from build123d import *

# Parameters (mm, degrees)
F1_DEPTH = 3.2


with BuildPart() as f1:
    # F0 (on Front) → F1 (new body)
    with BuildSketch(Plane.XZ):
        with BuildLine():
            Line((30.850063, 1.770954), (-56.149937, 1.770954))
            ThreePointArc((-56.149937, 1.770954), (-58.271257, 0.892275), (-59.149937, -1.229046))
            Line((-59.149937, -1.229046), (-59.149937, -16.129046))
            ThreePointArc((-59.149937, -16.129046), (-58.271257, -18.250366), (-56.149937, -19.129046))
            Line((-56.149937, -19.129046), (30.850063, -19.129046))
            ThreePointArc((30.850063, -19.129046), (32.971384, -18.250366), (33.850063, -16.129046))
            Line((33.850063, -16.129046), (33.850063, -1.229046))
            ThreePointArc((33.850063, -1.229046), (32.971384, 0.892275), (30.850063, 1.770954))
        make_face()
        Polygon((-56.249937, -16.129046), (-56.249937, -14.429046), (23.450063, -14.429046), (23.450063, -12.929046), (28.450063, -12.929046), (28.450063, -14.429046), (30.950063, -14.429046), (30.950063, -16.129046), align=None, mode=Mode.SUBTRACT)
    extrude(amount=F1_DEPTH)


solid = f1.part
The listing builds one solid part. Answer for the finished solid, in the listing's coordinates (mm). A direction names the side the tool comes from. Coordinates: 2 decimals unless noted, no trailing zeros. Order: outer loops, then holes, each group sorted by start corner. A loop starts at its lowest first (then second) coordinate and runs counter-clockwise, first axis right, second up. Notation, with made-up numbers: M 30.5,62 L 63.5,62 A11 ccw 63.5,72 Z; hole C 89,0.25 d7. An arc over 180 degrees is marked long. Use CSV: the item, a comma, the result in double quotes.
Q1. Section A-A (x = -26) is taken. Determine the outline of the cut face in (y, z).
Here are the results:
outline,"M -3.2,-19.13 L 0,-19.13 L 0,-16.13 L -3.2,-16.13 Z; M -3.2,-14.43 L 0,-14.43 L 0,1.77 L -3.2,1.77 Z"
Q2. A tool of negligible diameter and unlimited length cuts with its end or side. For faces 1 (the flat face through (30, -2, -14.429)), 2 (the flat face through (33.85, -2, -9)), from which of +Z, -Z, +X, -X, +Y, -Y can it reach the whole face along a straight path? Write none if from no direction.
Here are the results:
face 1,"+Y, -Y"
face 2,"+Z, -Z, +X, +Y, -Y"
Q3. Straight lines are drawn through the part: L1, parallel to Z at x = 22, y = -0.95; L2, parallel to X at y = -1.2, z = -15.75; L3, parallel to X at y = -2.3, z = -14.25. For each, find the intervals that lie inside material, in ascending order.
Here are the results:
L1,"-19.13 to -16.13, -14.43 to 1.77"
L2,"-59.15 to -56.25, 30.95 to 33.85"
L3,"-59.15 to 23.45, 28.45 to 33.85"
Q4. Section B-B (y = -0.65) is taken. Determine the outline of the cut face in (x, z), then the cut area to 3 significant figures.
Here are the results:
outline,"M -59.15,-16.13 A3 ccw -56.15,-19.13 L 30.85,-19.13 A3 ccw 33.85,-16.13 L 33.85,-1.23 A3 ccw 30.85,1.77 L -56.15,1.77 A3 ccw -59.15,-1.23 Z; hole M -56.25,-16.13 L 30.95,-16.13 L 30.95,-14.43 L 28.45,-14.43 L 28.45,-12.93 L 23.45,-12.93 L 23.45,-14.43 L -56.25,-14.43 Z"
area,"1,780 mm2"
Q5. Section C-C (x = 27) is taken. Determine the outline of the cut face in (y, z).
Here are the results:
outline,"M -3.2,-19.13 L 0,-19.13 L 0,-16.13 L -3.2,-16.13 Z; M -3.2,-12.93 L 0,-12.93 L 0,1.77 L -3.2,1.77 Z"
Q6. Determine the mould class of faces 3 (the cylindrical face through (-58.29, -1.58, -18.23)), 4 (the flat face through (23.45, -2, -14)), 5 (the flat face through (-12, -2, 1.771)) for opening direction X: pulls with the +X half, pulls with the -X half, needs draft (parallel to the pull), parting line crosses it, or undercut.
Here are the results:
face 3,"pulls with the -X half"
face 4,"undercut"
face 5,"needs draft"
